Geometry check sheet. Reference: the model listing, model coordinates, mm. Face numbers are marked on the shaded views. A direction names the side the tool comes from. Round coordinates to 2 decimals unless told otherwise and drop trailing zeros. Loops run counter-clockwise (first coordinate to the right, second up) from the corner with the lowest first, then second, coordinate; pieces in that order, holes last. Notation, with made-up numbers: M 10,44.25 L 15,44.25 A12 cw 15,52.25 Z; hole C 4,71 d7. An arc over 180 degrees is marked long. Write item = value, one per line.
from build123d import *

# Parameters (mm, degrees)
BOSS_EXTRUDE1_DEPTH  = 20
SKETCH3_R            = 1.25
SKETCH3_R_2          = 5
SKETCH3_R_3          = 2.25
CUT_EXTRUDE1_DEPTH   = 40
CUT_EXTRUDE2_DEPTH   = 40
MIRROR2_COPY_1_DEPTH = 40
BOSS_EXTRUDE3_DEPTH  = 2.5
SKETCH6_W            = 107.318523781
SKETCH6_H            = 36.59372062
CUT_EXTRUDE3_DEPTH   = 25
SKETCH7_W            = 103.85031415
SKETCH7_H            = 15.718097745
CUT_EXTRUDE4_DEPTH   = 50
SKETCH8_W            = 102.493521885
SKETCH8_H            = 23.554949116
CUT_EXTRUDE5_DEPTH   = 50
SKETCH9_W            = 100
SKETCH9_H            = 5
CUT_EXTRUDE6_DEPTH   = 50
FILLET1_R            = 400
FILLET2_R            = 10
FILLET3_START        = -2.629939755
FILLET3_DEPTH        = 5.259872573
FILLET3_START_2      = -10.0000001
FILLET3_2_DEPTH      = 20.0000001
FILLET3_START_3      = -176
FILLET3_3_DEPTH      = 156
SKETCH10_R           = 2
CUT_EXTRUDE7_DEPTH   = 10


with BuildPart() as part:
    # Sketch2 → Boss-Extrude1 (new, symmetric)
    with BuildSketch(Plane.XY):
        Polygon((0, 0), (200, 0), (200, 10), (-200, 10), (-200, 0), align=None)
    extrude(amount=BOSS_EXTRUDE1_DEPTH, both=True)

    # Sketch3 → Cut-Extrude1 (cut)
    with BuildSketch(Plane(origin=(0, 10, 0), x_dir=(1, 0, 0), z_dir=(0, 1, 0))):
        with Locations(Location((-4, 15.491933385, 0), (0, 0, 180))):
            Circle(SKETCH3_R)
        with Locations(Location((15.416407865, -4.281865077, 0), (0, 0, 180))):
            Circle(SKETCH3_R)
        with Locations(Location((-11.416407865, -11.210068308, 0), (0, 0, 180))):
            Circle(SKETCH3_R)
        with Locations(Location((0, 0, 0), (0, 0, 180))):
            Circle(SKETCH3_R_2)
        with Locations(Location((-190, 0, 0), (0, 0, 180))):
            Circle(SKETCH3_R_3)
        with Locations(Location((190, 0, 0), (0, 0, 270))):
            Circle(SKETCH3_R_3)
    extrude(amount=-CUT_EXTRUDE1_DEPTH, mode=Mode.SUBTRACT)

    # Sketch4 → Cut-Extrude2 (cut)
    with BuildSketch(Plane(origin=(0, 10, 0), x_dir=(1, 0, 0), z_dir=(0, 1, 0))):
        Polygon((-205.682411406, 30.266574236), (-25, 30.266574236), (-25, 20), (-200, 10), (-205.682411406, 10), align=None)
    cut_extrude2 = extrude(amount=-CUT_EXTRUDE2_DEPTH, mode=Mode.SUBTRACT)

    # Mirror1: Cut-Extrude2 across plane
    add(cut_extrude2.mirror(Plane(origin=(0, 0, 0), x_dir=(0, 0, 1), z_dir=(1, 0, 0))), mode=Mode.SUBTRACT)

    # Mirror2: Cut-Extrude2 across plane
    add(cut_extrude2.mirror(Plane.XY), mode=Mode.SUBTRACT)

    # Mirror2 copy 1 sketch → Mirror2 copy 1 (cut)
    with BuildSketch(Plane(origin=(0, 10, 0), x_dir=(-1, 0, 0), z_dir=(0, 1, 0))):
        Polygon((-205.682411406, 30.266574236), (-25, 30.266574236), (-25, 20), (-200, 10), (-205.682411406, 10), align=None)
    extrude(amount=-MIRROR2_COPY_1_DEPTH, mode=Mode.SUBTRACT)

    # Sketch5 → Boss-Extrude3 (add, symmetric)
    with BuildSketch(Plane.XY):
        Polygon((-175, 10), (-20, 10), (-130, 20), align=None)
    boss_extrude3 = extrude(amount=BOSS_EXTRUDE3_DEPTH, both=True)

    # Mirror3: Boss-Extrude3 across plane
    add(boss_extrude3.mirror(Plane(origin=(0, 0, 0), x_dir=(0, 0, 1), z_dir=(1, 0, 0))))

    # Sketch6 → Cut-Extrude3 (cut, symmetric)
    with BuildSketch(Plane.XY):
        with Locations((153.659261891, 18.29686031)):
            Rectangle(SKETCH6_W, SKETCH6_H)
    extrude(amount=CUT_EXTRUDE3_DEPTH, both=True, mode=Mode.SUBTRACT)

    # Sketch7 → Cut-Extrude4 (cut)
    with BuildSketch(Plane.XY):
        with Locations((51.925157075, 12.859048873)):
            Rectangle(SKETCH7_W, SKETCH7_H)
    extrude(amount=-CUT_EXTRUDE4_DEPTH, mode=Mode.SUBTRACT)

    # Sketch8 → Cut-Extrude5 (cut)
    with BuildSketch(Plane.XY):
        with Locations((51.246760943, 11.777474558)):
            Rectangle(SKETCH8_W, SKETCH8_H)
    extrude(amount=CUT_EXTRUDE5_DEPTH, mode=Mode.SUBTRACT)

    # Sketch9 → Cut-Extrude6 (cut)
    with BuildSketch(Plane.XY):
        with Locations((-50, 2.5)):
            Rectangle(SKETCH9_W, SKETCH9_H)
    extrude(amount=CUT_EXTRUDE6_DEPTH, mode=Mode.SUBTRACT)

    # Fillet1
    # the kernel refuses this fillet: 400 mm, written as the material it takes off along each edge
    with BuildSketch(Plane(origin=(-130, 20, 155.27904863), x_dir=(-0.9761870601839527, -0.21693045781865625, 0), z_dir=(0, 0, -1))) as fillet1_piece_1:
        with BuildLine():
            CenterArc((63.556611275, -399.618802355), FILLET1_R, 92.501596354, 15.221640262)
            Line((-58.21114592, -18.603562098), (-60.646501064, -10.983257293))
            Line((-60.646501064, -10.983257293), (-2.435355144, 7.620304805))
            Line((-2.435355144, 7.620304805), (0, 8))
            ThreePointArc((0, 8), (23.048861143, 8), (45.748544507, 7.992376047))
            Line((45.748544507, 7.992376047), (46.097722286, 0))
        make_face()
    extrude(amount=310.558097261, mode=Mode.SUBTRACT)

    # Fillet2
    fillet2_edges = [part.edges().sort_by_distance(p)[0] for p in [
        (-200, 5, -10),
        (-200, 5, 10),
    ]]
    fillet(fillet2_edges, radius=FILLET2_R)

    # Fillet3: read off the stored shape, not the designer's step
    # Fillet3 outline → Fillet3 (add)
    with BuildSketch(Plane.XY.offset(FILLET3_START)):
        with BuildLine():
            Line((-20, 10), (-69.139353351, 14.467213941))
            ThreePointArc((-69.139353351, 14.467213941), (-122.218339331, 15.75425111), (-175.000186885, 9.999966956))
            Line((-175.000186885, 9.999966956), (-20, 10))
        make_face()
    extrude(amount=FILLET3_DEPTH)

    # Fillet3 2 outline → Fillet3 2 (add)
    with BuildSketch(Plane.XY.offset(FILLET3_START_2)):
        with BuildLine():
            Line((-20, 10), (-69.139353351, 14.467213941))
            ThreePointArc((-69.139353351, 14.467213941), (-122.218339331, 15.75425111), (-175.000186885, 9.999966956))
            Line((-175.000186885, 9.999966956), (-20, 10))
        make_face()
    extrude(amount=FILLET3_2_DEPTH)

    # Fillet3 3 outline → Fillet3 3 (cut)
    with BuildSketch(Plane.YZ.offset(FILLET3_START_3)):
        with BuildLine():
            ThreePointArc((10, 10), (11.726129638, 5.213307923), (16.109978945, 2.629936129))
            Line((16.109978945, 2.629936129), (18, 2.273471232))
            Line((18, 2.273471232), (18, 10))
            Line((18, 10), (10, 10))
        make_face()
        with BuildLine():
            Line((18, -10.0000001), (18, -2.273470992))
            Line((18, -2.273470992), (16.109978046, -2.629936298))
            ThreePointArc((16.109978046, -2.629936298), (11.726129346, -5.213308275), (10, -10))
            Line((10, -10), (18, -10.0000001))
        make_face()
    extrude(amount=FILLET3_3_DEPTH, mode=Mode.SUBTRACT)

    # Sketch10 → Cut-Extrude7 (cut)
    with BuildSketch(Plane.XZ):
        with Locations(Location((-80, 13.351433229, 0), (0, 0, 270))):
            Circle(SKETCH10_R)
        with Locations(Location((80, -13.351433229, 0), (0, 0, 270))):
            Circle(SKETCH10_R)
    extrude(amount=-CUT_EXTRUDE7_DEPTH, mode=Mode.SUBTRACT)


solid = part.part
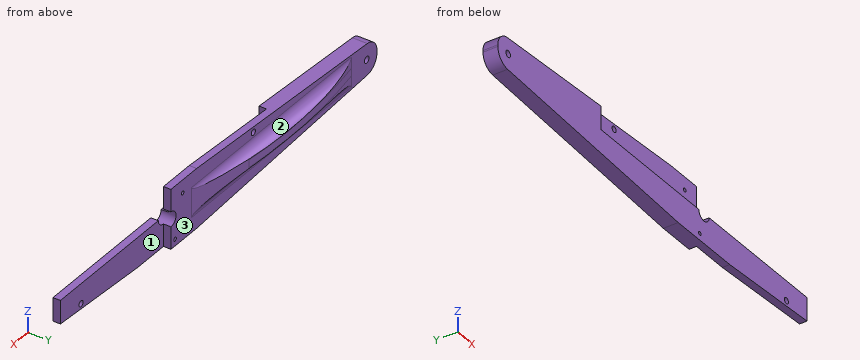
(1) Depth check by flat-ended pin: pin 1 Ø2 at (x, y) = (-156.5, 13.5) entering from -Z; pin 2 Ø22 at (x, z) = (59.5, -15) entering from +Y; pin 3 Ø3 at (x, z) = (-11.42, 11.21) entering from +Y; pin 4 Ø3 at (x, z) = (-4, -15.49) entering from -Y. Enter the tip coordinate at first touch or a pass-through.
Result set:
pin_1 = -4.41
pin_2 = 5
pin_3 = 10
pin_4 = 0
(2) Material ranges on line 1 along Z through (x, y) = (-4, 8); line 2 along Y through (x, z) = (-1, -6.5); line 3 along Y through (x, z) = (-166.5, 0.5), recorded low to high. Write a range as from..to.
Result set:
line_1 = -20..-16.74, -14.24..-3, 3..20
line_2 = 0..10
line_3 = 0..11.41
(3) Sectioned sample at B-B on x = 45. Record the cut outline in (y, z).
Result set:
outline = M 0,-18.86 L 5,-18.86 L 5,0 L 0,0 Z
(4) Sectioned sample at A-A on x = -74.5. Record the cut outline in (y, z), then the cut area to 3 significant figures.
Result set:
outline = M 0,-17.17 L 10,-17.17 L 10,-10 A7.5 cw 14.92,-2.96 L 14.92,2.96 A7.5 cw 10,10 L 10,17.17 L 5,17.17 L 5,0 L 0,0 Z
area = 306 mm2
(5) Tool access check on the marked faces 1, 2 and 3. Record the directions out of +Z, -Z, +X, -X, +Y, -Y that give a thin tool (end or side, any length) a straight path to the whole face; none if there is none.
Result set:
face_1 = +Z, -Z, +X, +Y
face_2 = +Z, +X, -X, +Y
face_3 = +Y
